from build123d import *

# Parameters (mm, degrees)
SKETCH1_R               = 35
BOSS_EXTRUDE1_DEPTH     = 10
SKETCH2_R               = 1.15
CUT_EXTRUDE1_DEPTH      = 3
BOSS_EXTRUDE2_DEPTH     = 5
CUT_EXTRUDE3_DEPTH      = 52.720402164
CUT_EXTRUDE3_DEPTH_BACK = 52.720402164
SKETCH12_R              = 1.15
CUT_EXTRUDE4_START      = -8
CUT_EXTRUDE4_OUTLINE_R  = 1.15
CUT_EXTRUDE4_DEPTH      = 9
SKETCH14_R              = 22.5
CUT_EXTRUDE5_DEPTH      = 2
SKETCH15_R              = 1.25
CUT_EXTRUDE6_DEPTH      = 6
CUT_EXTRUDE7_START      = -1
CUT_EXTRUDE7_DEPTH      = 6


with BuildPart() as part:
    # Sketch1 → Boss-Extrude1 (new body)
    with BuildSketch(Plane(origin=(0, 0, 0), x_dir=(1, 0, 0), z_dir=(0, 1, 0))):
        with Locations(Location((0, 0, 0), (0, 0, 270))):
            Circle(SKETCH1_R)
    extrude(amount=BOSS_EXTRUDE1_DEPTH)

    # Sketch2 → Cut-Extrude1 (cut)
    with BuildSketch(Plane(origin=(0, 10, 0), x_dir=(1, 0, 0), z_dir=(0, 1, 0))):
        Polygon((-21.773504548, -7.743563281), (-21.773504548, -11), (30.226495452, -11), (30.226495452, -8), (25.226495452, -8), (25.226495452, 8), (30.226495452, 8), (30.226495452, 11), (-21.773504548, 11), (-21.773504548, 8), (-16.773504548, 8), (-16.773504548, -7.743563281), align=None)
        with Locations(Location((-19.480382443, -5.75, 0), (0, 0, 270))):
            Circle(SKETCH2_R)
        with Locations(Location((-19.480382443, 5.75, 0), (0, 0, 270))):
            Circle(SKETCH2_R)
        with Locations(Location((27.993107277, 5.75, 0), (0, 0, 270))):
            Circle(SKETCH2_R)
        with Locations(Location((27.993107277, -5.75, 0), (0, 0, 270))):
            Circle(SKETCH2_R)
    extrude(amount=-CUT_EXTRUDE1_DEPTH, mode=Mode.SUBTRACT)

    # Sketch3 → Boss-Extrude2 (add)
    with BuildSketch(Plane(origin=(0, 10, 0), x_dir=(1, 0, 0), z_dir=(0, 1, 0))):
        with BuildLine():
            Line((30.726495452, 11.5), (30.726495452, 5.5))
            Line((30.726495452, 5.5), (34.565155865, 5.5))
            ThreePointArc((34.565155865, 5.5), (-35, 0), (34.565155865, -5.5))
            Line((34.565155865, -5.5), (30.726495452, -5.5))
            Line((30.726495452, -5.5), (30.726495452, -11.5))
            Line((30.726495452, -11.5), (28.788018341, -11.5))
            ThreePointArc((28.788018341, -11.5), (-31, 0), (28.788018341, 11.5))
            Line((28.788018341, 11.5), (30.726495452, 11.5))
        make_face()
    extrude(amount=BOSS_EXTRUDE2_DEPTH)

    # Sketch12 → Cut-Extrude3 (cut, two sides: drawn at the far end of the back side and taken through both)
    with BuildSketch(Plane.XZ.offset(-CUT_EXTRUDE3_DEPTH_BACK)):
        with Locations(Location((-23.334523779, 23.334523779, 0), (0, 0, 270))):
            Circle(SKETCH12_R)
        with Locations(Location((23.334523779, 23.334523779, 0), (0, 0, 270))):
            Circle(SKETCH12_R)
        with Locations(Location((23.334523779, -23.334523779, 0), (0, 0, 270))):
            Circle(SKETCH12_R)
        with Locations(Location((-23.334523779, -23.334523779, 0), (0, 0, 270))):
            Circle(SKETCH12_R)
    extrude(amount=CUT_EXTRUDE3_DEPTH + CUT_EXTRUDE3_DEPTH_BACK, mode=Mode.SUBTRACT)

    # Cut-Extrude4: read off the stored shape, not the designer's step
    # Cut-Extrude4 outline → Cut-Extrude4 (cut)
    # profile 1 of 4: a face of its own
    with BuildSketch(Plane.XZ.offset(CUT_EXTRUDE4_START)):
        with BuildLine():
            ThreePointArc((-25.816694029, -23.632568828), (-24.748737342, -24.748737342), (-23.632568828, -25.816694029))
            ThreePointArc((-23.632568828, -25.816694029), (-21.566756826, -21.566756826), (-25.816694029, -23.632568828))
        make_face()
        with Locations((-23.334523779, -23.334523779)):
            Circle(CUT_EXTRUDE4_OUTLINE_R, mode=Mode.SUBTRACT)
    # profile 2 of 4: a face of its own
    with BuildSketch(Plane.XZ.offset(CUT_EXTRUDE4_START)):
        with BuildLine():
            ThreePointArc((25.816694029, -23.632568828), (21.566756826, -21.566756826), (23.632568828, -25.816694029))
            ThreePointArc((23.632568828, -25.816694029), (24.748737342, -24.748737342), (25.816694029, -23.632568828))
        make_face()
        with Locations((23.334523779, -23.334523779)):
            Circle(CUT_EXTRUDE4_OUTLINE_R, mode=Mode.SUBTRACT)
    # profile 3 of 4: a face of its own
    with BuildSketch(Plane.XZ.offset(CUT_EXTRUDE4_START)):
        with BuildLine():
            ThreePointArc((-23.632568828, 25.816694029), (-24.748737342, 24.748737342), (-25.816694029, 23.632568828))
            ThreePointArc((-25.816694029, 23.632568828), (-21.566756826, 21.566756826), (-23.632568828, 25.816694029))
        make_face()
        with Locations((-23.334523779, 23.334523779)):
            Circle(CUT_EXTRUDE4_OUTLINE_R, mode=Mode.SUBTRACT)
    # profile 4 of 4: a face of its own
    with BuildSketch(Plane.XZ.offset(CUT_EXTRUDE4_START)):
        with BuildLine():
            ThreePointArc((25.816694029, 23.632568828), (24.748737342, 24.748737342), (23.632568828, 25.816694029))
            ThreePointArc((23.632568828, 25.816694029), (21.566756826, 21.566756826), (25.816694029, 23.632568828))
        make_face()
        with Locations((23.334523779, 23.334523779)):
            Circle(CUT_EXTRUDE4_OUTLINE_R, mode=Mode.SUBTRACT)
    extrude(amount=CUT_EXTRUDE4_DEPTH, mode=Mode.SUBTRACT)

    # Fillet2: read off the stored shape, not the designer's step
    # Fillet2 outline → Fillet2 (revolve, cut)
    with BuildSketch(Plane.XY):
        with BuildLine():
            ThreePointArc((35, 8), (32.656854249, 2.343145751), (27, 0))
            Line((27, 0), (35, 0))
            Line((35, 0), (35, 8))
        make_face()
    revolve(axis=Axis((0, 0, 0), (0, 1, 0)), mode=Mode.SUBTRACT)

    # Sketch14 → Cut-Extrude5 (cut)
    with BuildSketch(Plane.XZ):
        with Locations(Location((0, 0, 0), (0, 0, 270))):
            Circle(SKETCH14_R)
    extrude(amount=-CUT_EXTRUDE5_DEPTH, mode=Mode.SUBTRACT)

    # Sketch15 → Cut-Extrude6 (cut)
    with BuildSketch(Plane(origin=(0, 10, 0), x_dir=(1, 0, 0), z_dir=(0, 1, 0))):
        with Locations(Location((-10.25, 13, 0), (0, 0, 270))):
            Circle(SKETCH15_R)
        with Locations(Location((-10.25, -13, 0), (0, 0, 270))):
            Circle(SKETCH15_R)
        with Locations(Location((10.25, 13, 0), (0, 0, 270))):
            Circle(SKETCH15_R)
        with Locations(Location((10.25, -13, 0), (0, 0, 270))):
            Circle(SKETCH15_R)
    extrude(amount=-CUT_EXTRUDE6_DEPTH, mode=Mode.SUBTRACT)

    # Cut-Extrude7: read off the stored shape, not the designer's step
    # Cut-Extrude7 outline → Cut-Extrude7 (cut)
    with BuildSketch(Plane(origin=(0, 10, 0), x_dir=(1, 0, 0), z_dir=(0, 1, 0)).offset(CUT_EXTRUDE7_START)):
        with BuildLine():
            ThreePointArc((34.565155865, -5.5), (35, 0), (34.565155865, 5.5))
            Line((34.565155865, 5.5), (30.726495452, 5.5))
            Line((30.726495452, 5.5), (30.726495452, -5.5))
            Line((30.726495452, -5.5), (34.565155865, -5.5))
        make_face()
    extrude(amount=CUT_EXTRUDE7_DEPTH, mode=Mode.SUBTRACT)


solid = part.part
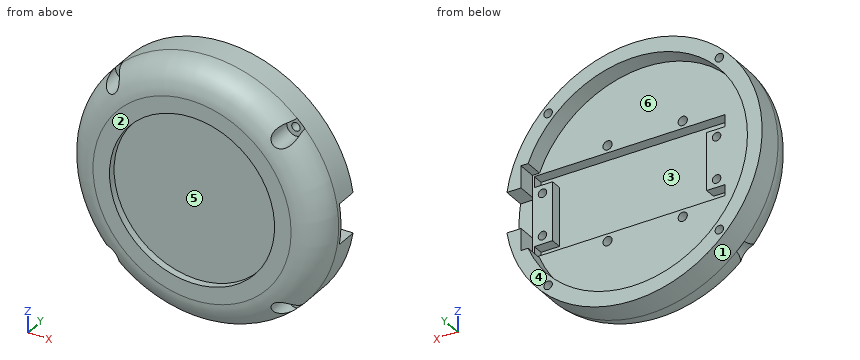
Geometry: final body of the model. Coordinates: model frame, mm. Face numbers are marked on the shaded views. A direction names the side the tool comes from. Give positions to 0.01 mm unless a question says otherwise; leave off trailing zeros. Write each loop counter-clockwise with the first axis right and the second up, starting at its lowest first coordinate (ties: lowest second). Pieces come first, ordered by that corner, then holes.
(1) Mould query, pull axis X, two halves, no side actions, for the marked faces 1, 2 and 3. Classes: released by +X, released by -X, zero draft, split by the parting line, or undercut.
(2) Access query for the marked faces 4, 5 and 6. Directions: +Z, -Z, +X, -X, +Y, -Y. A direction counts if a zero-diameter tool reaches every point of the face in a straight line with its end or side. Return the directions, or none.
(3) First-contact query: P1, Ø8, axis at x = -28, y = 9, coming from the -Z side; P2, Ø2.5, axis at y = 13, z = -8.5, coming from the -X side; P3, Ø2, axis at y = 10, z = 24, coming from the +X side. Flat tips, straight axial feed; report the tip coordinate or a pass-through.
(4) Cut plane B-B, the plane y = 5. Return loops of the section in (x, z).
(5) Ray query, line 1 (Z direction, x = 0, y = 12.2); line 2 (X direction, y = 9.75, z = 22.5); line 3 (Y direction, x = -3, z = 8.5). Return the intervals inside material, ascending.
(6) Cut plane A-A, the plane y = 13.5. Return loops of the section in (x, z).
Values follow:
1. face 1: split by the parting line
1. face 2: zero draft
1. face 3: undercut
2. face 4: +Z, -Z, +X, -X, +Y
2. face 5: -Y
2. face 6: +Y
3. P1: stops at z = -25.48
3. P2: stops at x = -34.24
3. P3: stops at x = 26.38
4. outline: (-25.78, -22.8) arc R2.5 cw (long way) to (-22.8, -25.78) arc R34.42 ccw to (22.8, -25.78) arc R2.5 cw (long way) to (25.78, -22.8) arc R34.42 ccw to (25.78, 22.8) arc R2.5 cw (long way) to (22.8, 25.78) arc R34.42 ccw to (-22.8, 25.78) arc R2.5 cw (long way) to (-25.78, 22.8) arc R34.42 ccw to start; hole circle Ø2.5 at (-10.25, -13); hole circle Ø2.5 at (-10.25, 13); hole circle Ø2.5 at (10.25, -13); hole circle Ø2.5 at (10.25, 13)
5. line 1: z = -35 to -31, 31 to 35
5. line 2: x = -26.81 to -24.13, -22.54 to 22.54, 24.13 to 26.81
5. line 3: y = 2 to 7
6. outline: (28.79, -11.5) arc R31 cw (long way) to (28.79, 11.5) - (30.73, 11.5) - (30.73, 5.5) - (34.57, 5.5) arc R35 ccw (long way) to (34.57, -5.5) - (30.73, -5.5) - (30.73, -11.5) - close; hole circle Ø2.3 at (-23.33, -23.33); hole circle Ø2.3 at (-23.33, 23.33); hole circle Ø2.3 at (23.33, -23.33); hole circle Ø2.3 at (23.33, 23.33)
